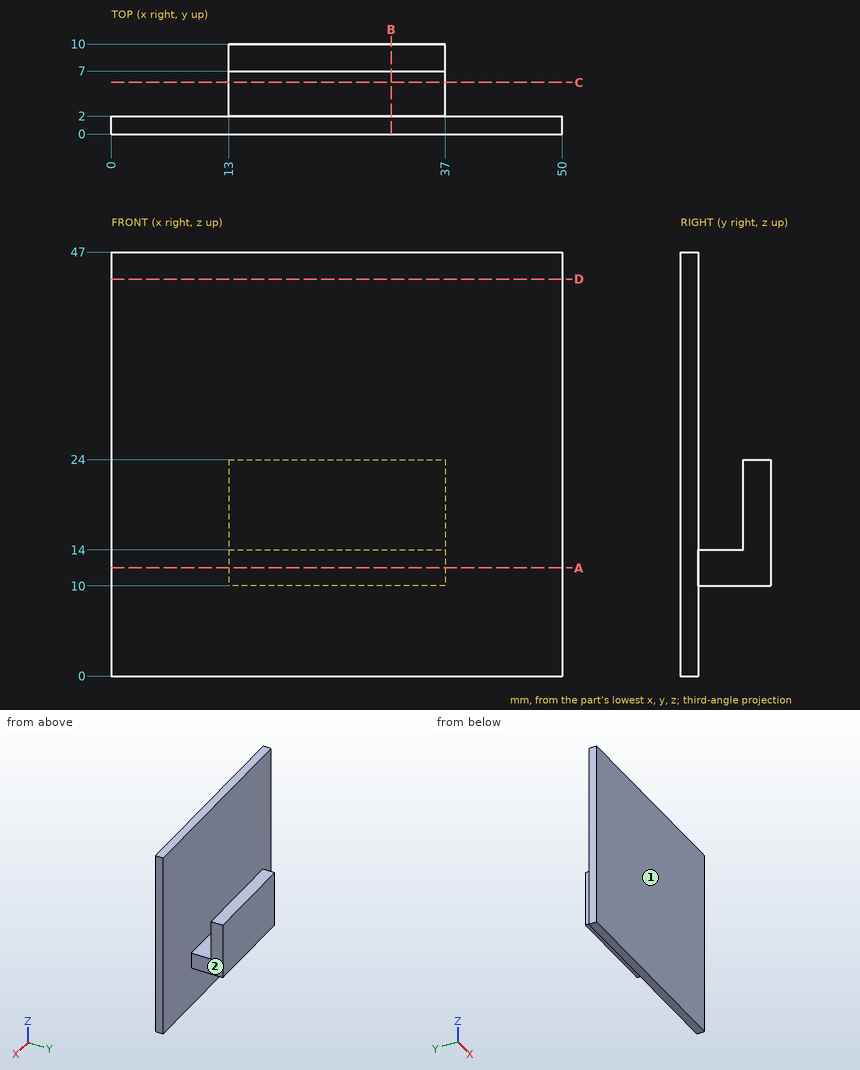
Verification items for this drawing (mm, ordinates from the low corner). A direction names the side the tool comes from. Give positions to 0.01 mm unless a question says otherwise; leave off trailing zeros. Write each loop counter-clockwise with the first axis right and the second up, starting at its lowest first coordinate (ties: lowest second). Pieces come first, ordered by that corner, then holes.
1) Section check A-A, the plane z = 12. Record the boundary of the cut face in (x, y).
2) Section check C-C, the plane y = 5.75. Record the boundary of the cut face in (x, z), and give its area (3 significant figures).
3) Section check D-D, the plane z = 44. Record the boundary of the cut face in (x, y).
4) Section check B-B, the plane x = 31. Record the boundary of the cut face in (y, z), and give its area (3 significant figures).
5) Access from +Z, -Z, +X, -X, +Y, -Y to the whole of each face (thin tool, end or side, straight path). Record for the marked faces 1 and 2.
6) Material ranges on L1, parallel to Y at x = 27.5, z = 14.5; L2, parallel to Y at x = 43, z = 22; L3, parallel to Z at x = 21.5, y = 6, recorded low to high.
7) Gauge pin test, flat ends, axial feed: pin 1 (4 mm diameter, centred on y = 5.5, z = 17.5, fed in from -X); pin 2 (4 mm diameter, centred on x = 19.5, y = 4.5, fed in from +Z); pin 3 (1.5 mm diameter, centred on y = 7.5, z = 13, fed in from +X). Record the tip position at first contact, or that the pin passes through.
Computed:
1. outline: (0, 0) - (50, 0) - (50, 2) - (37, 2) - (37, 10) - (13, 10) - (13, 2) - (0, 2) - close
2. outline: (13, 10) - (37, 10) - (37, 14) - (13, 14) - close
2. area: 96.0 mm2
3. outline: (0, 0) - (50, 0) - (50, 2) - (0, 2) - close
4. outline: (0, 0) - (2, 0) - (2, 10) - (10, 10) - (10, 24) - (7, 24) - (7, 14) - (2, 14) - (2, 47) - (0, 47) - close
4. area: 156 mm2
5. face 1: +Z, -Z, +X, -X, -Y
5. face 2: +Z, -Z, +X, +Y
6. L1: y = 0 to 2, 7 to 10
6. L2: y = 0 to 2
6. L3: z = 10 to 14
7. pin 1: stops at x = 13
7. pin 2: stops at z = 14
7. pin 3: stops at x = 37
